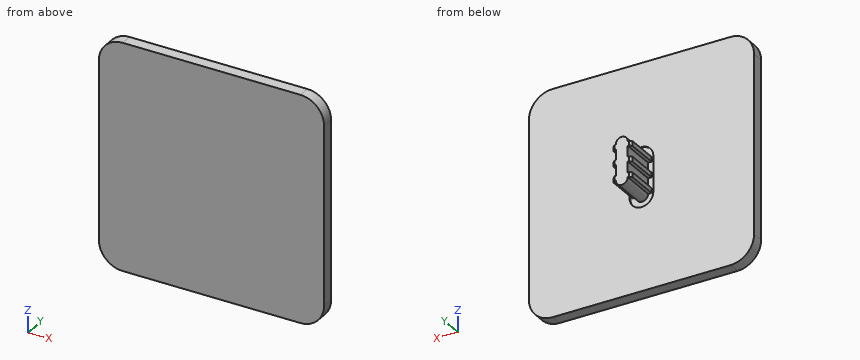
```python
from build123d import *

# Parameters (mm, degrees)
BOSS_EXTRUDE1_DEPTH             = 5
CUT_EXTRUDE1_DEPTH              = 0.5
BOSS_EXTRUDE2_DEPTH             = 14
BOSS_EXTRUDE2_DIRECTION_2_REACH = 7
CHAMFER2_SIZE                   = 1


with BuildPart() as part:
    # Sketch1 → Boss-Extrude1 (new body)
    with BuildSketch(Plane(origin=(0, 0, 0), x_dir=(1, 0, 0), z_dir=(0, 1, 0))):
        with BuildLine():
            Line((10, 0), (85, 0))
            ThreePointArc((85, 0), (92.071067812, 2.928932188), (95, 10))
            Line((95, 10), (95, 85))
            ThreePointArc((95, 85), (92.071067812, 92.071067812), (85, 95))
            Line((85, 95), (10, 95))
            ThreePointArc((10, 95), (2.928932188, 92.071067812), (0, 85))
            Line((0, 85), (0, 10))
            ThreePointArc((0, 10), (2.928932188, 2.928932188), (10, 0))
        make_face()
    extrude(amount=BOSS_EXTRUDE1_DEPTH)

    # Sketch4 → Cut-Extrude1 (cut)
    with BuildSketch(Plane(origin=(0, 5, 0), x_dir=(1, 0, 0), z_dir=(0, 1, 0))):
        with BuildLine():
            Line((52.5, 55), (52.5, 40))
            ThreePointArc((52.5, 40), (47.5, 35), (42.5, 40))
            Line((42.5, 40), (42.5, 55))
            ThreePointArc((42.5, 55), (47.5, 60), (52.5, 55))
        make_face()
    extrude(amount=-CUT_EXTRUDE1_DEPTH, mode=Mode.SUBTRACT)

    # Sketch3 → Boss-Extrude2 (add)
    with BuildSketch(Plane(origin=(0, 5, 0), x_dir=(1, 0, 0), z_dir=(0, 1, 0))):
        with BuildLine():
            Line((45, 53.002509929), (45, 48.502509929))
            Line((45, 48.502509929), (43.5, 48.502509929))
            Line((43.5, 48.502509929), (43.5, 46.502509929))
            Line((43.5, 46.502509929), (45, 46.502509929))
            Line((45, 46.502509929), (45, 42.002509929))
            Line((45, 42.002509929), (43.5, 42.002509929))
            Line((43.5, 42.002509929), (43.5, 40.002509929))
            Line((43.5, 40.002509929), (45, 40.002509929))
            ThreePointArc((45, 40.002509929), (47.5, 37.502509929), (50, 40.002509929))
            Line((50, 40.002509929), (51.5, 40.002509929))
            Line((51.5, 40.002509929), (51.5, 42.002509929))
            Line((51.5, 42.002509929), (50, 42.002509929))
            Line((50, 42.002509929), (50, 46.502509929))
            Line((50, 46.502509929), (51.5, 46.502509929))
            Line((51.5, 46.502509929), (51.5, 48.502509929))
            Line((51.5, 48.502509929), (50, 48.502509929))
            Line((50, 48.502509929), (50, 53.002509929))
            Line((50, 53.002509929), (51.5, 53.002509929))
            Line((51.5, 53.002509929), (51.5, 55.002509929))
            Line((51.5, 55.002509929), (50, 55.002509929))
            ThreePointArc((50, 55.002509929), (47.5, 57.502509929), (45, 55.002509929))
            Line((45, 55.002509929), (43.5, 55.002509929))
            Line((43.5, 55.002509929), (43.5, 53.002509929))
            Line((43.5, 53.002509929), (45, 53.002509929))
        make_face()
    extrude(amount=BOSS_EXTRUDE2_DEPTH)

    # Sketch3 → Boss-Extrude2 direction 2 (add, up to next)
    with BuildSketch(Plane(origin=(0, 5, 0), x_dir=(1, 0, 0), z_dir=(0, 1, 0)), mode=Mode.PRIVATE) as boss_extrude2_direction_2_sk1:
        with BuildLine():
            Line((45, 53.002509929), (45, 48.502509929))
            Line((45, 48.502509929), (43.5, 48.502509929))
            Line((43.5, 48.502509929), (43.5, 46.502509929))
            Line((43.5, 46.502509929), (45, 46.502509929))
            Line((45, 46.502509929), (45, 42.002509929))
            Line((45, 42.002509929), (43.5, 42.002509929))
            Line((43.5, 42.002509929), (43.5, 40.002509929))
            Line((43.5, 40.002509929), (45, 40.002509929))
            ThreePointArc((45, 40.002509929), (47.5, 37.502509929), (50, 40.002509929))
            Line((50, 40.002509929), (51.5, 40.002509929))
            Line((51.5, 40.002509929), (51.5, 42.002509929))
            Line((51.5, 42.002509929), (50, 42.002509929))
            Line((50, 42.002509929), (50, 46.502509929))
            Line((50, 46.502509929), (51.5, 46.502509929))
            Line((51.5, 46.502509929), (51.5, 48.502509929))
            Line((51.5, 48.502509929), (50, 48.502509929))
            Line((50, 48.502509929), (50, 53.002509929))
            Line((50, 53.002509929), (51.5, 53.002509929))
            Line((51.5, 53.002509929), (51.5, 55.002509929))
            Line((51.5, 55.002509929), (50, 55.002509929))
            ThreePointArc((50, 55.002509929), (47.5, 57.502509929), (45, 55.002509929))
            Line((45, 55.002509929), (43.5, 55.002509929))
            Line((43.5, 55.002509929), (43.5, 53.002509929))
            Line((43.5, 53.002509929), (45, 53.002509929))
        make_face()
    boss_extrude2_direction_2_tool1 = extrude(boss_extrude2_direction_2_sk1.sketch, amount=-BOSS_EXTRUDE2_DIRECTION_2_REACH, mode=Mode.PRIVATE) - part.part
    add(boss_extrude2_direction_2_tool1.solids().sort_by_distance((47.5, 5, -47.50251))[0])

    # Chamfer2
    chamfer2_edges = [part.edges().sort_by_distance(p)[0] for p in [
        (43.5, 19, -47.502509929),
        (43.5, 19, -41.002509929),
        (51.5, 19, -41.002509929),
        (51.5, 19, -47.502509929),
        (51.5, 19, -54.002509929),
        (43.5, 19, -54.002509929),
    ]]
    chamfer(chamfer2_edges, length=CHAMFER2_SIZE)


solid = part.part
```
For this review, take the finished solid that the model builds, in its own axes (mm). Round coordinates to 2 decimals unless told otherwise and drop trailing zeros. Write each loop counter-clockwise with the first axis right and the second up, starting at its lowest first coordinate (ties: lowest second). Pieces come first, ordered by that corner, then holes. Notation, with made-up numbers: (67.25, 80) -> (79.25, 80) arc R20 cw to (79.25, 88) -> close; hole circle Ø10 at (56.5, 63.25). An arc over 180 degrees is marked (long way). One line per question, with ' | ' between items. Start each with the question number.
1) For pin 1 Ø1.3 at (y, z) = (11, -44) entering from -X; pin 2 Ø1.2 at (x, y) = (44, 9.5) entering from -Z; pin 3 Ø3 at (x, z) = (19.5, -31) entering from +Y; pin 4 Ø3 at (x, z) = (44.5, -32) entering from -Y, all flat-tipped, find the tip position at first contact; note any pin that passes through.
2) Wall thickness on line 1 along Y through (x, z) = (8.5, -46.5); line 2 along X through (y, z) = (15.25, -51); line 3 along X through (y, z) = (6.5, -54): over which ranges is each line inside the solid? List them lowest first.
3) Add section B-B (x = 47.5). Write out the cut boundary in (y, z), and give its area (4 significant figures).
4) Add section A-A (y = 15.75). Write out the cut boundary in (x, z).
5) Add section D-D (x = 79.5). Write out the cut boundary in (y, z), and give its area (3 significant figures).
6) Add section C-C (z = -79). Write out the cut boundary in (x, y).
Reported:
1) pin 1: stops at x = 45 | pin 2: stops at z = -55 | pin 3: stops at y = 5 | pin 4: stops at y = 0
2) line 1: y = 0 to 5 | line 2: x = 45 to 50 | line 3: x = 43.5 to 51.5
3) outline: (0, -95) -> (5, -95) -> (5, -60) -> (4.5, -60) -> (4.5, -57.5) -> (19, -57.5) -> (19, -37.5) -> (4.5, -37.5) -> (4.5, -35) -> (5, -35) -> (5, 0) -> (0, 0) -> close | area: 752.5 mm²
4) outline: (43.5, -55) -> (45, -55) arc R2.5 ccw to (50, -55) -> (51.5, -55) -> (51.5, -53) -> (50, -53) -> (50, -48.5) -> (51.5, -48.5) -> (51.5, -46.5) -> (50, -46.5) -> (50, -42) -> (51.5, -42) -> (51.5, -40) -> (50, -40) arc R2.5 ccw to (45, -40) -> (43.5, -40) -> (43.5, -42) -> (45, -42) -> (45, -46.5) -> (43.5, -46.5) -> (43.5, -48.5) -> (45, -48.5) -> (45, -53) -> (43.5, -53) -> close
5) outline: (0, -95) -> (5, -95) -> (5, 0) -> (0, 0) -> close | area: 475 mm²
6) outline: (0, 0) -> (95, 0) -> (95, 5) -> (0, 5) -> close
